The model under review builds one solid part; all positions refer to its coordinate system, in mm. Face numbers are marked on the shaded views. A direction names the side the tool comes from. Round coordinates to 2 decimals unless told otherwise and drop trailing zeros. Write each loop counter-clockwise with the first axis right and the second up, starting at its lowest first coordinate (ties: lowest second). Pieces come first, ordered by that corner, then holes. Notation, with made-up numbers: (17.25, 28) -> (43.25, 28) arc R18 cw to (43.25, 58) -> close; hole circle Ø10 at (67.5, -1.75). An arc over 180 degrees is marked (long way). Answer in a Markdown table with one row per item. Add a question column.
```python
from build123d import *

# Parameters (mm, degrees)
F0_R = 16.677954


with BuildPart() as f2:
    # F0 (on Top) → F2 (revolve)
    with BuildSketch(Plane.XY):
        Polygon((46.619876, -35.406111), (56.74863, 14.373538), (24.144508, 53.329619), (-26.640921, 52.12741), (-57.365193, 11.672198), (-44.892304, -37.572418), (1.385405, -58.524236), align=None)
        Circle(F0_R, mode=Mode.SUBTRACT)
    revolve(axis=Axis((76.640435, 3.132816, 0), (0, -1, 0)))


solid = f2.part
```
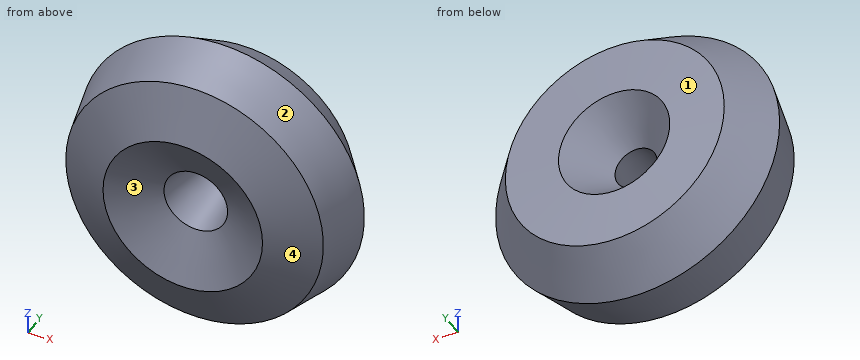
1. For L1, parallel to X at y = -10, z = 13; L2, parallel to X at y = 48, z = -38; L3, parallel to X at y = 41, z = -25, list the stretches that pass through material, from the lowest coordinate up.
2. Tool access review of the marked faces 1 and 2: name each direction out of +Z, -Z, +X, -X, +Y, -Y from which nothing blocks a thin tool from reaching the whole face with its end or side.
3. Insertion check: pin 1 Ø1 at (y, z) = (-44, 16.5) entering from +X; pin 2 Ø1.5 at (x, z) = (66, 35) entering from -Y; pin 3 Ø12 at (x, y) = (119.5, 25.5) entering from +Z; pin 4 Ø12 at (x, z) = (182, -93.5) entering from -Y. Each pin has a flat end and moves straight along its axis. Give the tip position at first contact, or say it passes through.
4. Add section B-B on y = 31.5. Write out the cut boundary in (x, z).
5. Add section A-A on z = 0. Write out the cut boundary in (x, y).
6. Mouldability with a two-part tool opening along X and no side actions: class the marked faces 3 and 4 as pulls with the +X half, pulls with the -X half, needs draft (parallel to the pull), parting line crosses it, or undercut.
7. Add section C-C on x = 92. State how many separate pieces and enclosed holes the cut face has, plus the area to 3 significant figures.
Filled in:
| question | item | result |
|---|---|---|
| 1 | L1 | -51.22 to -12.4, 14.7 to 55.46, 97.82 to 138.58, 165.68 to 204.5 |
| 1 | L2 | -22.76 to 47.26, 106.02 to 176.04 |
| 1 | L3 | -32.26 to 42.67, 110.61 to 185.54 |
| 2 | face 1 | +Y |
| 2 | face 2 | -Y |
| 3 | pin 1 | x = 183.82 |
| 3 | pin 2 | y = -39.14 |
| 3 | pin 3 | z = 121.1 |
| 3 | pin 4 | through |
| 4 | outline | circle Ø237.89 at (76.64, 0); hole circle Ø68.45 at (76.64, 0) |
| 5 | outline | (-57.37, 11.67) -> (-44.89, -37.57) -> (1.39, -58.52) -> (46.62, -35.41) -> (56.75, 14.37) -> (24.14, 53.33) -> (-26.64, 52.13) -> close; (96.53, 14.37) -> (106.66, -35.41) -> (151.9, -58.52) -> (198.17, -37.57) -> (210.65, 11.67) -> (179.92, 52.13) -> (129.14, 53.33) -> close; hole circle Ø33.36 at (0, 0); hole circle Ø33.36 at (153.28, 0) |
| 6 | face 3 | undercut |
| 6 | face 4 | parting line crosses it |
| 7 | separate pieces | 2 |
| 7 | enclosed holes | 2 |
| 7 | area | 17,700 mm² |
